The model under review builds one solid part; all positions refer to its coordinate system, in mm. Face numbers are marked on the shaded views. Coordinates: 2 decimals unless noted, no trailing zeros. Write each loop counter-clockwise with the first axis right and the second up, starting at its lowest first coordinate (ties: lowest second). Pieces come first, ordered by that corner, then holes. Notation, with made-up numbers: M 41,85.25 L 48,85.25 A27 ccw 48,116.25 Z; hole C 20,70.25 d10. An arc over 180 degrees is marked long. Answer as CSV lines item,"result". Start each with the question number.
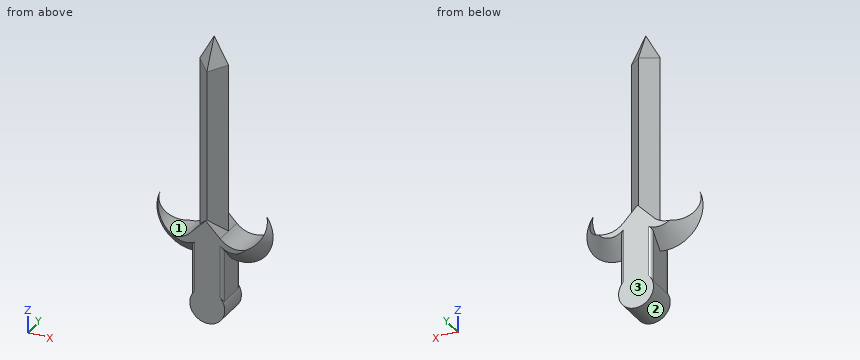
from build123d import *

# Parameters (mm, degrees)
F1_DEPTH    = 10
F2_SIZE     = 4.99999
F3_T1_DEPTH = 67.4287295288
F4_DEPTH    = 10
F5_T4_ANGLE = 302.1740734605
F5_T9_ANGLE = 359.64
F6_T4_ANGLE = 359.64
F6_T9_ANGLE = 302.1740734605
F7_R        = 1


# Not quite as in the source:
# - a fillet or chamfer that OpenCascade refuses, or shapes differently, is made with other operations: its cross-section is extruded or revolved along the edge and cut away or added
# - a fillet or chamfer is up to 0.001 mm smaller than in the source, because OpenCascade refuses the exact size


with BuildPart() as f1:
    # F0 (on Front) → F1 (new body)
    with BuildSketch(Plane.XZ):
        Polygon((35.3119149804, 10.4430096801), (39.7443734109, 5.9087900445), (39.7443734109, 57.9162985086), (35.3119149804, 65.8947229385), (30.8794565499, 57.9162985086), (30.8794565499, 5.9087900445), align=None)
    extrude(amount=F1_DEPTH)

    # F2 (size 5 in the source; OpenCascade refuses exactly that, so slightly less here)
    f2_edges = [f1.edges().sort_by_distance(p)[0] for p in [
        (37.528144, -10, 61.905511),
        (37.528144, 0, 61.905511),
        (33.095686, -10, 61.905511),
        (33.095686, 0, 61.905511),
    ]]
    chamfer(f2_edges, length=F2_SIZE)

    # F3: chamfer of 5 on 4 edges, made by hand

    # F3_s2 → F3_t1 (cut)
    with BuildSketch(Plane.XY.offset(-6.9496248953)):
        Polygon((30.8794565499, -5), (35.8794565499, 0), (30.8794565499, 0), align=None)
        Polygon((30.8794565499, -5), (35.8794565499, -10), (30.8794565499, -10), align=None)
        Polygon((34.7443734109, -10), (39.7443734109, -5), (39.7443734109, -10), align=None)
        Polygon((34.7443734109, 0), (39.7443734109, -5), (39.7443734109, 0), align=None)
    extrude(amount=F3_T1_DEPTH, mode=Mode.SUBTRACT)

    # F0 (on Front) → F4 (join)
    with BuildSketch(Plane.XZ):
        with BuildLine():
            ThreePointArc((51.5925973184, 13.3139307646), (48.6483872163, 4.8435179428), (39.7443734109, 5.9087900445))
            Line((39.7443734109, 5.9087900445), (35.3119149804, 10.4430096801))
            Line((35.3119149804, 10.4430096801), (30.8794565499, 5.9087900445))
            ThreePointArc((30.8794565499, 5.9087900445), (21.5650677315, 4.2615226747), (18.7640711665, 13.2962195203))
            ThreePointArc((18.7640711665, 13.2962195203), (19.9563786111, 1.6237063121), (30.8794565499, -2.6606291067))
            Line((30.8794565499, -2.6606291067), (30.8794565499, -13.8895222917))
            ThreePointArc((30.8794565499, -13.8895222917), (35.755161196, -21.5906926023), (40.6308658421, -13.8895222917))
            Line((40.6308658421, -13.8895222917), (40.6308658421, -2.3651318625))
            ThreePointArc((40.6308658421, -2.3651318625), (51.65255991, 1.6006300969), (51.5925973184, 13.3139307646))
        make_face()
    extrude(amount=F4_DEPTH)

    # F5: chamfer of 5 on 2 edges, made by hand


with BuildPart() as f5_tool2:
    # F5_s3 → F5_t4 (revolve)
    with BuildSketch(Plane(origin=(9.3560149059, 0, -9.9565277283), x_dir=(0, 1, 0), z_dir=(0.6847887183, 0, -0.728741663))):
        Polygon((-10, 33.1289388428), (-5, 38.1289388428), (-10, 38.1289388428), align=None)
    revolve(axis=Axis((28.9307170955, -10, 8.4375560791), (0, -1, 0)), revolution_arc=F5_T4_ANGLE)

    split(bisect_by=Plane.YZ.offset(30.8794565499), keep=Keep.BOTTOM)


with BuildPart() as f1_1:
    add(f1.part)

    # F5_t1: cut F5_tool2
    add(f5_tool2.part, mode=Mode.SUBTRACT)


with BuildPart() as f5_tool7:
    # F5_s8 → F5_t9 (revolve)
    with BuildSketch(Plane(origin=(12.756533571, 0, -16.3882307622), x_dir=(0, 1, 0), z_dir=(-0.6142445443, 0, 0.7891157328))):
        Polygon((-5, -28.604545656), (-10, -33.604545656), (-10, -28.604545656), align=None)
    revolve(axis=Axis((43.3362013883, -10, 7.4148609054), (0, -1, 0)), revolution_arc=F5_T9_ANGLE)

    split(bisect_by=Plane.YZ.offset(40.6308658421), keep=Keep.TOP)


with BuildPart() as f1_2:
    add(f1_1.part)

    # F5_t6: cut F5_tool7
    add(f5_tool7.part, mode=Mode.SUBTRACT)

    # F6: chamfer of 5 on 2 edges, made by hand


with BuildPart() as f6_tool2:
    # F6_s3 → F6_t4 (revolve)
    with BuildSketch(Plane(origin=(12.756533571, 0, -16.3882307622), x_dir=(0, 1, 0), z_dir=(-0.6142445443, 0, 0.7891157328))):
        Polygon((-5, -28.604545656), (0, -33.604545656), (0, -28.604545656), align=None)
    revolve(axis=Axis((43.3362013883, 0, 7.4148609054), (0, -1, 0)), revolution_arc=F6_T4_ANGLE)

    split(bisect_by=Plane.YZ.offset(40.6308658421), keep=Keep.TOP)


with BuildPart() as f1_3:
    add(f1_2.part)

    # F6_t1: cut F6_tool2
    add(f6_tool2.part, mode=Mode.SUBTRACT)


with BuildPart() as f6_tool7:
    # F6_s8 → F6_t9 (revolve)
    with BuildSketch(Plane(origin=(9.3560149059, 0, -9.9565277283), x_dir=(0, 1, 0), z_dir=(0.6847887183, 0, -0.728741663))):
        Polygon((-5, 38.1289388428), (0, 33.1289388428), (0, 38.1289388428), align=None)
    revolve(axis=Axis((28.9307170955, 0, 8.4375560791), (0, -1, 0)), revolution_arc=F6_T9_ANGLE)

    split(bisect_by=Plane.YZ.offset(30.8794565499), keep=Keep.BOTTOM)


with BuildPart() as f1_4:
    add(f1_3.part)

    # F6_t6: cut F6_tool7
    add(f6_tool7.part, mode=Mode.SUBTRACT)

    # F7
    f7_edges = [f1_4.edges().sort_by_distance(p)[0] for p in [
        (40.630866, 0, -5.426826),
        (30.879457, 0, -5.704655),
        (40.630866, -10, -5.426826),
        (30.879457, -10, -5.704655),
    ]]
    fillet(f7_edges, radius=F7_R)


solid = f1_4.part
1) Take a section at B-B on z = 27. Give the boundary of the cut face in (x, y).
2) Clearance check with flat-ended pins moving along their axes: pin 1 Ø4 at (y, z) = (-1, -8.5) entering from +X; pin 2 Ø4 at (y, z) = (-3.5, -6.5) entering from -X; pin 3 Ø2 at (x, y) = (24, -8) entering from +Z. State where each tip first meets the part, or that it passes through.
3) Take a section at A-A on y = -2.5. Give the boundary of the cut face in (x, z).
4) To check wall thickness, follow line 1 (X direction, y = -5.75, z = -4); line 2 (X direction, y = -1.25, z = -16.5); line 3 (Y direction, x = 42, z = 1). State the ranges of each line that lie inside material, in increasing order. Write a range as [from, to].
5) Mouldability with a two-part tool opening along X and no side actions: class the marked faces 1, 2 and 3 as +X half, -X half, draft (parallel to the pull), parting line (faces both ways), or undercut.
6) Take a section at D-D on z = 8. Give the number of separate pieces and of enclosed holes in the cut face, and give its area (3 significant figures).
Results:
1,outline,"M 30.88,-5 L 35.31,-9.43 L 39.74,-5 L 35.31,-0.57 Z"
2,pin 1,"stops at x = 40.63"
2,pin 2,"stops at x = 30.88"
2,pin 3,"stops at z = 3.59"
3,outline,"M 21.04,4.61 A8.77 ccw 30.88,-0.11 L 30.88,-13.89 A5.39 ccw long 40.63,-13.89 L 40.63,0.26 A7.65 ccw 50.98,7.21 A7.15 cw 39.74,5.91 L 37.24,8.47 L 37.24,57.27 L 35.31,60.75 L 33.38,57.27 L 33.38,8.47 L 30.88,5.91 A7.15 cw Z"
4,line 1,"x = [30.88, 40.63]"
4,line 2,"x = [30.37, 41.14]"
4,line 3,"y = [-8.59, -1.41]"
5,face 1,"undercut"
5,face 2,"parting line"
5,face 3,"draft"
6,separate pieces,"3"
6,enclosed holes,"0"
6,area,"61.2 mm²"
